Check sheet for the modelled part. Datum: model origin and axes. Units: mm. A direction names the side the tool comes from. Coordinates: 2 decimals unless noted, no trailing zeros. Order: outer loops, then holes, each group sorted by start corner. A loop starts at its lowest first (then second) coordinate and runs counter-clockwise, first axis right, second up. Notation, with made-up numbers: M 82.25,-19 L 124.25,-19 A12 cw 124.25,-7 Z; hole C 41,-31.5 d5. An arc over 180 degrees is marked long. Answer in a Markdown table with one row per item. Add a question column.
from build123d import *

# Parameters (mm, degrees)
BOSS_EXTRU_2_DEPTH      = 2.15
ESQUISSE2_W             = 14.75
ESQUISSE2_H             = 13
BOSS_EXTRU_3_DEPTH      = 6.3
BOSS_EXTRU_4_DEPTH      = 7.5
ESQUISSE1_5_W           = 14.75
ESQUISSE1_5_H           = 13
BOSS_EXTRUDE1_DEPTH     = 13
CHAMFER1_SIZE           = 11
ESQUISSE3_R             = 1.6
ENL_V_MAT_EXTRU_1_DEPTH = 6.3
ENL_V_START             = -4.15
ESQUISSE11_R            = 3.75
ENL_V_MAT_EXTRU_2_DEPTH = 4.15
ESQUISSE12_W            = 14.75
ESQUISSE12_H            = 8.4
BOSS_EXTRU_5_DEPTH      = 5.5
ESQUISSE13_W            = 16.3
ESQUISSE13_H            = 7.2
BOSS_EXTRU_6_DEPTH      = 2
ESQUISSE14_W            = 7.5
ESQUISSE14_H            = 7.2
BOSS_EXTRU_7_DEPTH      = 2
ESQUISSE16_W            = 15.8
ESQUISSE16_H            = 6.7
ENL_V_MAT_EXTRU_3_DEPTH = 1.5
BOSS_EXTRU_9_DEPTH      = 5.9
BOSS_EXTRU_10_DEPTH     = 10.1
ESQUISSE20_W            = 8.967116883
ESQUISSE20_H            = 2.3
ENL_V_MAT_EXTRU_4_DEPTH = 10.1


with BuildPart() as part:
    # Esquisse1 → Boss.-Extru.2 (new body)
    with BuildSketch(Plane.XY):
        with BuildLine():
            Line((20.065642458, -7.091397664), (16.315642458, -7.091397664))
            Line((16.315642458, -7.091397664), (16.315642458, 0.408602336))
            Line((16.315642458, 0.408602336), (20.065642458, 0.408602336))
            ThreePointArc((20.065642458, 0.408602336), (23.815642458, -3.341397664), (20.065642458, -7.091397664))
        make_face()
    extrude(amount=BOSS_EXTRU_2_DEPTH)



with BuildPart() as body_2:
    # Esquisse2 → Boss.-Extru.3 (new body)
    with BuildSketch(Plane.XY):
        with Locations((8.940642458, -3.341397664)):
            Rectangle(ESQUISSE2_W, ESQUISSE2_H)
    extrude(amount=BOSS_EXTRU_3_DEPTH)


with BuildPart() as part_1:
    add(part.part)

    add(body_2.part)  # Boss.-Extru.4 merges body 2
    # Esquisse10 → Boss.-Extru.4 (add)
    with BuildSketch(Plane.XZ.offset(7.091397664)):
        Polygon((16.315642458, 6.287787974), (20.065642458, 2.15), (16.315642458, 2.15), align=None)
    extrude(amount=-BOSS_EXTRU_4_DEPTH)

    # Esquisse1_5 → Boss-Extrude1 (add)
    with BuildSketch(Plane.XY):
        with Locations((8.940642458, -3.003724395)):
            Rectangle(ESQUISSE1_5_W, ESQUISSE1_5_H)
    extrude(amount=-BOSS_EXTRUDE1_DEPTH)

    # Chamfer1
    chamfer1_edges = [part_1.edges().sort_by_distance(p)[0] for p in [
        (8.940642458, 3.496275605, -13),
    ]]
    chamfer(chamfer1_edges, length=CHAMFER1_SIZE)

    # Esquisse3 → Enl_v. mat.-Extru.1 (cut)
    with BuildSketch(Plane.XY):
        with Locations((-16.934357542, -3.341397664)):
            Circle(ESQUISSE3_R)
        with Locations(Location((20.065642458, -3.341397664, 0), (0, 0, 90))):
            Circle(ESQUISSE3_R)
    extrude(amount=ENL_V_MAT_EXTRU_1_DEPTH, mode=Mode.SUBTRACT)

    # Esquisse11 → Enl_v. mat.-Extru.2 (cut)
    with BuildSketch(Plane.XY.offset(6.3).offset(ENL_V_START)):
        with Locations((20.065642458, -3.341397664)):
            Circle(ESQUISSE11_R)
    extrude(amount=ENL_V_MAT_EXTRU_2_DEPTH, mode=Mode.SUBTRACT)

    # Esquisse12 → Boss.-Extru.5 (add)
    with BuildSketch(Plane.XY.offset(6.3)):
        with Locations((8.940642458, -3.341397664)):
            Rectangle(ESQUISSE12_W, ESQUISSE12_H)
    extrude(amount=BOSS_EXTRU_5_DEPTH)

    # Sym_trie15: part across plane


with BuildPart() as part_2:
    add(part_1.part)
    add(part_1.part.mirror(Plane(origin=(1.565642458, 3.158602336, 6.3), x_dir=(0, 0, 1), z_dir=(1, 0, 0))))

    # Esquisse13 → Boss.-Extru.6 (add)
    with BuildSketch(Plane.XY.offset(11.8)):
        with Locations((7.365642458, -3.341397664)):
            Rectangle(ESQUISSE13_W, ESQUISSE13_H)
    extrude(amount=BOSS_EXTRU_6_DEPTH)

    # Esquisse14 → Boss.-Extru.7 (add)
    with BuildSketch(Plane.XY.offset(11.8)):
        with Locations((-8.684357542, -3.341397664)):
            Rectangle(ESQUISSE14_W, ESQUISSE14_H)
    extrude(amount=BOSS_EXTRU_7_DEPTH)

    # Esquisse16 → Enl_v. mat.-Extru.3 (cut)
    with BuildSketch(Plane.XY.offset(13.8)):
        with Locations((7.365642458, -3.341397664)):
            Rectangle(ESQUISSE16_W, ESQUISSE16_H)
    extrude(amount=-ENL_V_MAT_EXTRU_3_DEPTH, mode=Mode.SUBTRACT)

    # Esquisse15 → R_volution14 (revolve)
    with BuildSketch(Plane.XY.offset(12.3)):
        with BuildLine():
            Line((14.537530361, -3.341397664), (8.093754555, -3.341397664))
            ThreePointArc((8.093754555, -3.341397664), (11.315642458, -6.563285567), (14.537530361, -3.341397664))
        make_face()
        with BuildLine():
            Line((-11.779153482, -3.341397664), (-5.589561602, -3.341397664))
            ThreePointArc((-5.589561602, -3.341397664), (-8.684357542, -6.436193604), (-11.779153482, -3.341397664))
        make_face()
    revolve(axis=Axis((-12.130427956, -3.341397664, 12.3), (1, 0, 0)))

    # Esquisse18 → Boss.-Extru.9 (add)
    with BuildSketch(Plane(origin=(0, 3.158602336, 0), x_dir=(1, 0, 0), z_dir=(0, 1, 0))):
        Polygon((6.615642458, -4.5), (6.615642458, -9.05), (-3.484357542, -9.05), (-3.484357542, -4.5), (-4.37348724, -4.5), (-4.37348724, -3.3), (7.451018627, -3.3), (7.451018627, -4.5), align=None)
    extrude(amount=BOSS_EXTRU_9_DEPTH)

    # Esquisse19 → Boss.-Extru.10 (add)
    with BuildSketch(Plane.ZY.offset(3.484357542)):
        Polygon((6.3, 0.858602336), (7.675, 3.158602336), (6.3, 3.158602336), align=None)
    extrude(amount=-BOSS_EXTRU_10_DEPTH)

    # Esquisse20 → Enl_v. mat.-Extru.4 (cut)
    with BuildSketch(Plane.XY.offset(6.3)):
        with Locations((1.525201642, 2.008602336)):
            Rectangle(ESQUISSE20_W, ESQUISSE20_H)
    extrude(amount=ENL_V_MAT_EXTRU_4_DEPTH, mode=Mode.SUBTRACT)


solid = part_2.part
1. Section check A-A on z = 8.25. Enter the section's corners in (x, y).
2. Section check C-C on y = 5.75. Enter the section's corners in (x, z), then the cut area to 3 significant figures.
3. Set-up check for faces 1 (the flat face through (2, 3.496, -1)), 2 (the flat face through (-8, 2, 6.3)), 3 (the flat face through (22, -3, 2.15)), 4 (the flat face through (-2, -3, 11.8)): record each of +Z, -Z, +X, -X, +Y, -Y from which the full face is reachable in a straight line by a thin tool's end or side.
4. Section check D-D on x = 12. Enter the section's corners in (y, z), then the cut area to 3 significant figures.
5. Release check for a two-part mould opening along Y. For faces 5 (the cylindrical face through (-13.185, -3.259, 3.73)), 6 (the cylindrical face through (-18.35, -2.6, 1.06)), 7 (the flat face through (18, -7.091, 2)), 8 (the cylindrical face through (23.815, -3.259, 1.06)) record: released by +Y, released by -Y, zero draft, split by the parting line, or undercut.
6. Scan lines: line 1 (X direction, y = 1.5, z = 6.5); line 2 (Y direction, x = 8.5, z = 10.25); line 3 (X direction, y = 2.5, z = 2.5). Record each from-to range of solid material in increasing order.
7. Go/stop test with flat-tipped pins: pin 1 Ø1.5 at (x, z) = (14, 11) entering from -Y; pin 2 Ø1 at (x, z) = (4.5, 12.5) entering from +Y; pin 3 Ø5 at (y, z) = (-7, -4.5) entering from -X. Record where each tip stops, or that it passes through.
8. Section check B-B on x = 19. Enter the section's corners in (y, z), then the cut area to 3 significant figures.
Result sheet:
| question | item | result |
|---|---|---|
| 1 | outline | M -13.18,-7.54 L 16.32,-7.54 L 16.32,0.86 L -13.18,0.86 Z; M -3.48,3.16 L 6.62,3.16 L 6.62,9.06 L -3.48,9.06 Z |
| 2 | outline | M -4.37,3.3 L 7.45,3.3 L 7.45,4.5 L 6.62,4.5 L 6.62,9.05 L -3.48,9.05 L -3.48,4.5 L -4.37,4.5 Z |
| 2 | area | 60.1 mm^2 |
| 3 | face 1 | -Z, +X, -X, +Y |
| 3 | face 2 | +Z, -X, +Y |
| 3 | face 3 | +Z, +X |
| 3 | face 4 | +Z |
| 4 | outline | M -9.84,0 L -9.5,0 L -9.5,-13 L -7.5,-13 L 3.5,-2 L 3.5,0 L 3.16,0 L 3.16,6.3 L 0.86,6.3 L 0.86,11.8 L 0.26,11.8 L 0.26,13.8 L 0.01,13.8 L 0.01,12.3 L -0.19,12.3 A3.15 ccw -6.49,12.3 L -6.69,12.3 L -6.69,13.8 L -6.94,13.8 L -6.94,11.8 L -7.54,11.8 L -7.54,6.3 L -9.84,6.3 Z |
| 4 | area | 257 mm^2 |
| 5 | face 5 | undercut |
| 5 | face 6 | undercut |
| 5 | face 7 | released by -Y |
| 5 | face 8 | split by the parting line |
| 6 | line 1 | -3.48 to -2.96, 6.01 to 6.62 |
| 6 | line 2 | -7.54 to 0.86 |
| 6 | line 3 | -13.18 to 16.32 |
| 7 | pin 1 | y = -7.54 |
| 7 | pin 2 | y = 0.26 |
| 7 | pin 3 | x = -13.18 |
| 8 | outline | M -7.09,0 L -4.53,0 L -4.53,2.15 L -6.94,2.15 L -6.94,3.33 L -7.09,3.33 Z; M -2.15,0 L 0.41,0 L 0.41,3.33 L 0.25,3.33 L 0.25,2.15 L -2.15,2.15 Z |
| 8 | area | 11.4 mm^2 |
